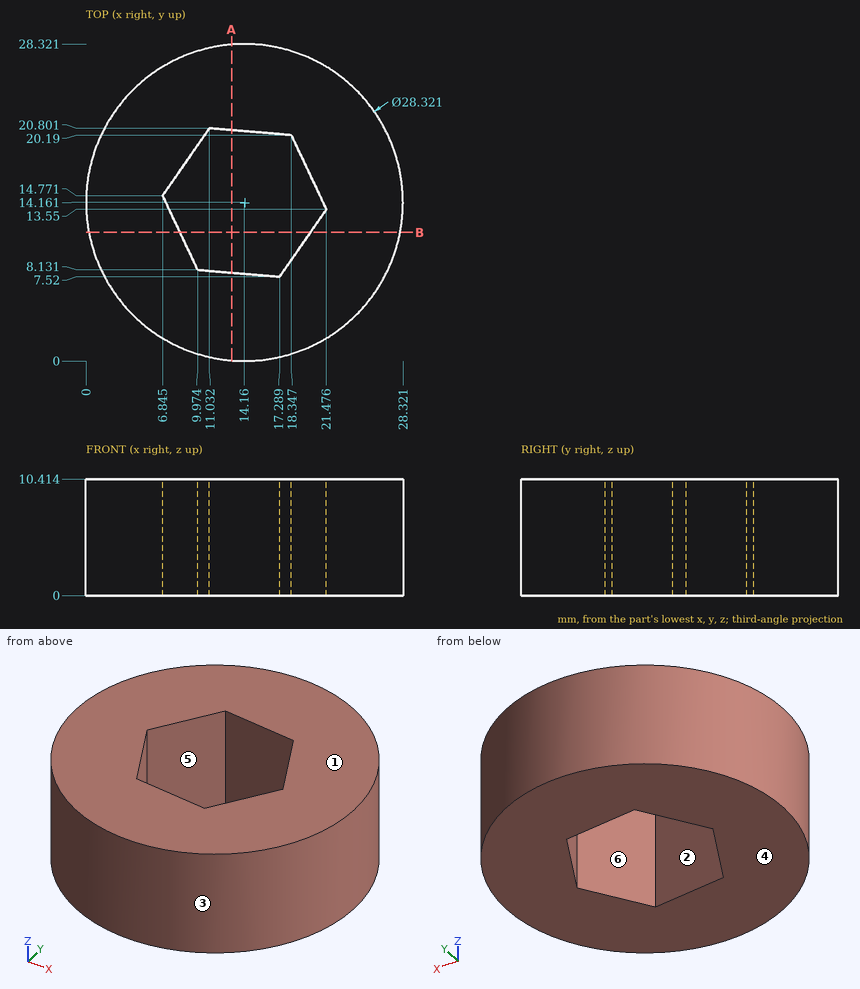
Drawing for the job (mm, zero at the part's lowest x, y, z). A direction names the side the tool comes from. Round coordinates to 2 decimals unless told otherwise and drop trailing zeros. Write each loop counter-clockwise with the first axis right and the second up, starting at its lowest first coordinate (ties: lowest second). Pieces come first, ordered by that corner, then holes. Notation, with made-up numbers: (33.5, 46) - (55.5, 46) arc R24 cw to (55.5, 74) - close; hole circle Ø4 at (50.5, 35.5). An arc over 180 degrees is marked (long way). Return JSON: item names as keys, results as strings. Group by question number.
Item 1: Mould opens along Y. For the marked faces 3, 4, 5 and 6 say: +Y half, -Y half, draft (parallel to the pull), parting line (faces both ways), or undercut.
Item 2: Band-saw the part on A-A on x = 13. List the corners of the cut face in (y, z) (1 decimal).
Item 3: Band-saw the part on B-B on y = 11.5. List the corners of the cut face in (x, z) (1 decimal).
Item 4: 3-axis set-ups, long thin cutter, end or side, ignore diameter. For the marked faces 1 and 2: which of +Z, -Z, +X, -X, +Y, -Y reach the whole face in a straight line?
Item 5: Flat gauge pin, fed straight in: pin 1 Ø2 at (y, z) = (17.5, 7.5) entering from +X. Where does the tip first touch, or does it go through?
Item 6: Probe probe 1 along Y at (x, z) = (17.75, 6.75) (1 decimal); probe 2 along Y at (x, z) = (9.25, 1) (1 decimal); probe 3 along X at (y, z) = (18.5, 4.5) (1 decimal). List the from-to ranges inside material, lowest first.
Resolved:
{
 "1": {"face 3": "parting line", "face 4": "draft", "face 5": "undercut", "face 6": "undercut"},
 "2": {"outline": "(0, 0) - (7.9, 0) - (7.9, 10.4) - (0, 10.4) - close; (20.6, 0) - (28.3, 0) - (28.3, 10.4) - (20.6, 10.4) - close"},
 "3": {"outline": "(0.3, 0) - (8.4, 0) - (8.4, 10.4) - (0.3, 10.4) - close; (20.1, 0) - (28.1, 0) - (28.1, 10.4) - (20.1, 10.4) - close"},
 "4": {"face 1": "+Z, +X, -X, +Y, -Y", "face 2": "+Z, -Z"},
 "5": {"pin 1": "stops at x = 28.13"},
 "6": {"probe 1": "y = 0.5 to 8.2, 20.2 to 27.9", "probe 2": "y = 0.9 to 9.7, 18.2 to 27.4", "probe 3": "x = 0.7 to 9.4, 19.1 to 27.6"}
}
